Geometry: final body of the model. Coordinates: model frame, mm. Face numbers are marked on the shaded views. Give positions to 0.01 mm unless a question says otherwise; leave off trailing zeros. Order: outer loops, then holes, each group sorted by start corner. A loop starts at its lowest first (then second) coordinate and runs counter-clockwise, first axis right, second up. Notation, with made-up numbers: (67, -11.75) -> (88, -11.75) arc R20 cw to (88, 22.25) -> close; hole circle Ø3 at (40, -16.75). An arc over 180 degrees is marked (long way). One line per item, written item: value. Start each with the question number.
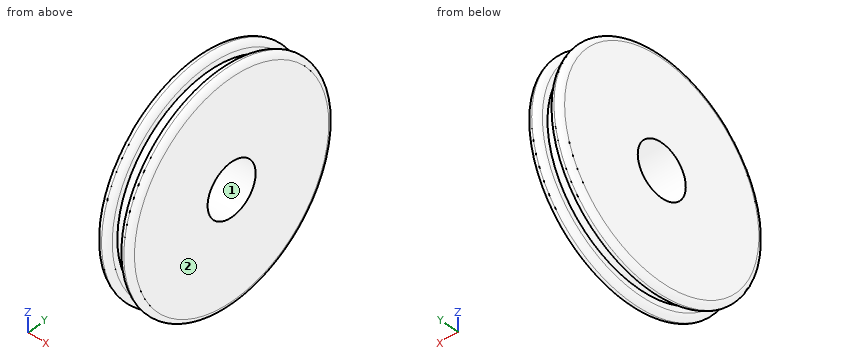
Autodesk Inventor part; units mm, degrees
ref_plane "YZ Plane" through (0, 0, 0) normal (1, 0, 0) x (0, 1, 0)
ref_plane "XZ Plane" through (0, 0, 0) normal (0, 1, 0) x (-1, 0, 0)
ref_plane "XY Plane" through (0, 0, 0) normal (0, 0, 1) x (1, 0, 0)
sketch "Boceto1" plane through (0, 0, 0) normal (1, 0, 0) x (0, 1, 0)
  circle A0 centre (0, 0) radius 10
  dimension "d2" = 20
extrude "Extrusión1" add sketch "Boceto1" along normal blind 3
ref_plane "Plano de trabajo1" through (1.5, 0, 0) normal (1, 0, 0) x (0, 0, -1)
sketch "Boceto2" plane through (1.5, 0, 0) normal (1, 0, 0) x (0, 0, -1)
  circle A0 centre (0, 0) radius 14.342
  circle A1 centre (0, 0) radius 9
  dimension "d3" = 18
extrude "Extrusión2" cut sketch "Boceto2" along normal blind 0.5 and the other way blind 0.5
fillet "Empalme1" radius 0.5 4 edges at (3, -10, 0) (2, -10, 0) (1, -10, 0) (0, -10, 0)
sketch "Boceto3" plane through (3, 0, 0) normal (1, 0, 0) x (0, 0, -1)
  circle A0 centre (0, 0) radius 2.35
  dimension "d9" = 4.7
extrude "Extrusión3" cut sketch "Boceto3" against normal blind 10
properties part number "rueda servo"
1. Draft query along Z for the marked faces 1 and 2. Return one class per face: pulls with the +Z half, pulls with the -Z half, needs draft (parallel to the pull), parting line crosses it, or undercut.
2. Material intervals for L1, parallel to Y at x = 1.55, z = 0; L2, parallel to X at y = 1, z = 9.25; L3, parallel to Y at x = 0.35, z = -3.25, sorted ascending. Write a range as [from, to].
3. Cut plane C-C, the plane x = 1.4. Return loops of the section in (y, z).
4. Pin query (flat end, axial travel): P1, Ø1.5, axis at x = 0.5, y = 7.5, coming from the +Z side. Return the tip coordinate at first contact, or that it passes through.
Answers follow:
1. face 1: undercut
1. face 2: needs draft
2. L1: y = [-9, -2.35], [2.35, 9]
2. L2: x = [0, 1], [2, 3]
2. L3: y = [-9.43, 9.43]
3. outline: circle Ø18 at (0, 0); hole circle Ø4.7 at (0, 0)
4. P1: stops at z = 7.38
